from build123d import *

# Parameters (mm, degrees)
F1_DEPTH = 50.8
F3_DEPTH = 25.4
F4_R     = 3.175
F5_DEPTH = 38.1


with BuildPart() as f1:
    # F0 (on Top) → F1 (new body)
    with BuildSketch(Plane.XY):
        Polygon((0, 8.89), (0, 0), (27.94, 0), (27.94, 8.89), (17.78, 8.89), (17.78, 17.78), (10.16, 17.78), (10.16, 8.89), align=None)
    extrude(amount=F1_DEPTH)

    # F2 (on face) → F3 (cut)
    with BuildSketch(Plane(origin=(10.16, 0, 0), x_dir=(0, -1, 0), z_dir=(-1, 0, 0))):
        Polygon((-17.78, 17.622068), (-8.89, 50.8), (-17.78, 50.8), align=None)
        with BuildLine():
            Line((-16.51, 0), (-10.16, 0))
            ThreePointArc((-10.16, 0), (-13.335, 3.175), (-16.51, 0))
        make_face()
    extrude(amount=-F3_DEPTH, mode=Mode.SUBTRACT)

    # F4 (on face) → F5 (cut)
    with BuildSketch(Plane(origin=(0, 0, 0), x_dir=(0, -1, 0), z_dir=(-1, 0, 0))):
        with Locations((-4.445, 44.45)):
            Circle(F4_R)
        with Locations((-4.445, 6.35)):
            Circle(F4_R)
    extrude(amount=-F5_DEPTH, mode=Mode.SUBTRACT)


solid = f1.part
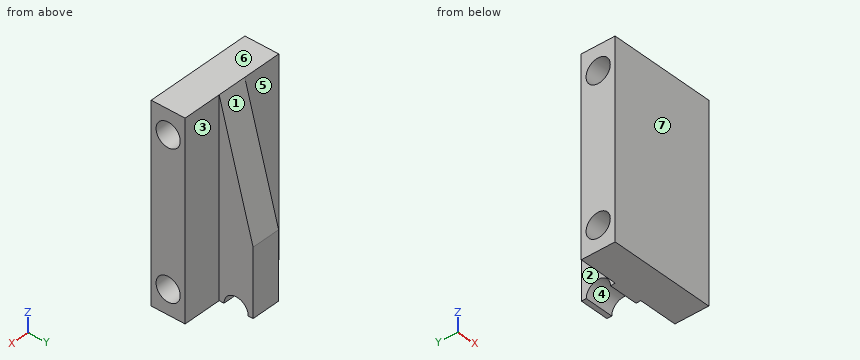
Can you work these out from the model? Positions are in its coordinate system, mm. Face numbers are marked on the shaded views. A direction names the side the tool comes from. Give positions to 0.01 mm unless a question says otherwise; leave off trailing zeros. Order: outer loops, then holes, each group sorted by start corner. A loop starts at its lowest first (then second) coordinate and runs counter-clockwise, first axis right, second up. Notation, with made-up numbers: M 26,85.25 L 84,85.25 A15 ccw 84,102.25 Z; hole C 5,46.25 d6. An arc over 180 degrees is marked long. Use one line per item in the form item = value.
Item 1: Will these pins go through, and if not, where does the flat tip stop? pin 1 Ø7 at (y, z) = (15.5, 16) entering from -X; pin 2 Ø2.5 at (y, z) = (13, 28) entering from +X; pin 3 Ø8 at (x, z) = (6.5, 34) entering from +Y.
Values follow:
pin_1 = 10.16
pin_2 = 17.78
pin_3 = 13.82
Item 2: Thinking about a two-plate mould opening in Y: for the marked faces 4, 5, 6 and 7, which applies, pulls with the +Y half, pulls with the -Y half, needs draft (parallel to the pull), parting line crosses it, or undercut?
Values follow:
face_4 = undercut
face_5 = pulls with the +Y half
face_6 = needs draft
face_7 = pulls with the -Y half
Item 3: If we section it at A-A, the plane z = 6.35: Write out the boundary of the cut face in (x, y), and give its area (3 significant figures).
Values follow:
outline = M 0,0 L 27.94,0 L 27.94,1.27 L 0,1.27 Z; M 0,7.62 L 27.94,7.62 L 27.94,8.89 L 17.78,8.89 L 17.78,17.78 L 10.16,17.78 L 10.16,8.89 L 0,8.89 Z
area = 139 mm^2
Item 4: If we section it at B-B, the plane x = 17.25: Write out the boundary of the cut face in (y, z) (3 decimals).
Values follow:
outline = M 0,0 L 10.16,0 A3.175 cw 16.51,0 L 17.78,0 L 17.78,17.622 L 8.89,50.8 L 0,50.8 Z; hole C 4.445,6.35 d6.35; hole C 4.445,44.45 d6.35
Item 5: For the marked faces 1, 2 and 3, which set-ups out of +Z, -Z, +X, -X, +Y, -Y let a thin tool reach every point of the face, with its end or its side?
Values follow:
face_1 = +Z, +X, -X, +Y
face_2 = +Z, -Z, -X, +Y
face_3 = +Z, -Z, +X, +Y
Item 6: If we section it at D-D, the plane z = 44.45: Write out the boundary of the cut face in (x, y), and give its area (3 significant figures).
Values follow:
outline = M 0,0 L 27.94,0 L 27.94,1.27 L 0,1.27 Z; M 0,7.62 L 27.94,7.62 L 27.94,8.89 L 17.78,8.89 L 17.78,10.59 L 10.16,10.59 L 10.16,8.89 L 0,8.89 Z
area = 83.9 mm^2
Item 7: If we section it at C-C, the plane z = 24.5: Write out the boundary of the cut face in (x, y).
Values follow:
outline = M 0,0 L 27.94,0 L 27.94,8.89 L 17.78,8.89 L 17.78,15.94 L 10.16,15.94 L 10.16,8.89 L 0,8.89 Z
Item 8: If I drill on line 1 along Z through (x, y) = (4.5, 7); line 2 along Z through (x, y) = (18.25, 6.5); line 3 along Y through (x, z) = (7, 29), over which ranges is the centre line in solid material (lowest first)? Write a range as [from, to].
Values follow:
line_1 = [0, 4.47], [8.23, 42.57], [46.33, 50.8]
line_2 = [0, 3.93], [8.77, 42.03], [46.87, 50.8]
line_3 = [0, 8.89]
